Geometry check sheet. Reference: the model listing, model coordinates, mm. A direction names the side the tool comes from. Coordinates: 2 decimals unless noted, no trailing zeros. Write each loop counter-clockwise with the first axis right and the second up, starting at its lowest first coordinate (ties: lowest second). Pieces come first, ordered by that corner, then holes. Notation, with made-up numbers: (-27.75, 75) -> (-1.75, 75) arc R27 ccw to (-1.75, 104) -> close; hole circle Ø10 at (-2.75, 64). An arc over 180 degrees is marked (long way). Answer in a Markdown table with one row per item. Add a question column.
Q1. Section check D-D, the plane x = 0. Count the separate pieces of the cut face and the enclosed holes in it, and give its area (3 significant figures).
Q2. Release check for a two-part mould opening along X. For faces 5 (the face through (-42.15, 250.51, 0.45)), 6 (the face through (0.49, 2.85, -41.99)), 7 (the face through (-1.69, 57.89, 33.87)) record: pulls with the +X half, pulls with the -X half, needs draft (parallel to the pull), parting line crosses it, or undercut.
Q3. Tool access check on faces 1 (the face through (0, 105, 75)), 2 (the face through (0, 22.5, 0)), 3 (the face through (7.067, 56.084, -25.354)), 4 (the face through (42.15, 136.72, 25.51)). Record the directions out of +Z, -Z, +X, -X, +Y, -Y that give a thin tool (end or side, any length) a straight path to the whole face; none if there is none.
Q4. Section check A-A, the plane y = 105. Record the boundary of the cut face in (x, z), and give its area (3 significant figures).
Q5. Thickness scan on line 1 (Y direction, x = 0, z = 32.75); line 2 (Y direction, x = -25, z = -16.5); line 3 (Z direction, x = 9.5, y = 99). Record the ranges inside material, lowest first.
Q6. Section check B-B, the plane y = 170.5. Record the boundary of the cut face in (x, z), and give its area (3 significant figures).
Q7. Gauge pin test, flat ends, axial feed: P1, Ø1, axis at x = -26, y = 241, coming from the -Z side; P2, Ø6, axis at x = -1, y = 132.5, coming from the +Z side; P3, Ø15.5, axis at x = 0, y = 45, coming from the +Z side; P4, Ø10, axis at x = -16, z = -50.5, coming from the -Y side. Record the tip position at first contact, or that the pin passes through.
Q8. Section check C-C, the plane x = -22. Record the boundary of the cut face in (y, z).
```python
from build123d import *

# Parameters (mm, degrees)
SKETCH2_W              = 90
SKETCH2_H              = 90
BOSS_EXTRUDE1_DEPTH    = 270
SKETCH3_W              = 45
SKETCH3_H              = 225
CUT_EXTRUDE1_DEPTH     = 289.140590684
SKETCH4_R              = 25
CRANK_SHAFT_HOLE_DEPTH = 90
SKETCH5_R              = 13
CUT_EXTRUDE3_DEPTH     = 90
CHAMFER1_SIZE          = 3
SKETCH6_R              = 17.5
BOSS_EXTRUDE2_DEPTH    = 30
FILLET1_R              = 10


with BuildPart() as part:
    # Sketch2 → Boss-Extrude1 (new body)
    with BuildSketch(Plane(origin=(0, 0, 0), x_dir=(1, 0, 0), z_dir=(0, 1, 0))):
        Rectangle(SKETCH2_W, SKETCH2_H)
    extrude(amount=BOSS_EXTRUDE1_DEPTH)

    # Sketch3 → Cut-Extrude1 (cut, through all)
    with BuildSketch(Plane(origin=(45, 0, 0), x_dir=(0, 0, -1), z_dir=(1, 0, 0))):
        with Locations((0, 135)):
            Rectangle(SKETCH3_W, SKETCH3_H)
    extrude(amount=-CUT_EXTRUDE1_DEPTH, mode=Mode.SUBTRACT)

    # Sketch4 → Crank shaft hole (cut)
    with BuildSketch(Plane.XY.offset(45)):
        with Locations((0, 170.5)):
            Circle(SKETCH4_R)
    extrude(amount=-CRANK_SHAFT_HOLE_DEPTH, mode=Mode.SUBTRACT)

    # Sketch5 → Cut-Extrude3 (cut)
    with BuildSketch(Plane.XY.offset(45)):
        with Locations((0, 45)):
            Circle(SKETCH5_R)
    extrude(amount=-CUT_EXTRUDE3_DEPTH, mode=Mode.SUBTRACT)

    # Chamfer1
    chamfer1_edges = [part.edges().sort_by_distance(p)[0] for p in [
        (-13, 45, 22.5),
        (-13, 45, -45),
        (-13, 45, -22.5),
        (-13, 45, 45),
    ]]
    chamfer(chamfer1_edges, length=CHAMFER1_SIZE)

    # Sketch6 → Boss-Extrude2 (add)
    with BuildSketch(Plane.XY.offset(45)):
        with Locations(Location((0, 105, 0), (0, 0, 180))):
            Circle(SKETCH6_R)
    boss_extrude2 = extrude(amount=BOSS_EXTRUDE2_DEPTH)

    # Mirror1: Boss-Extrude2 across plane
    add(boss_extrude2.mirror(Plane.XY))

    # Fillet1
    fillet1_edges = [part.edges().sort_by_distance(p)[0] for p in [
        (-45, 270, 0),
        (0, 270, 45),
        (-45, 135, 22.5),
        (-45, 247.5, 0),
        (-45, 135, -22.5),
        (-45, 22.5, 0),
        (45, 135, 22.5),
        (45, 22.5, 0),
        (45, 135, -22.5),
        (45, 247.5, 0),
        (45, 270, 0),
        (0, 0, 45),
        (-45, 0, 0),
        (0, 0, -45),
        (45, 0, 0),
        (45, 135, 45),
        (-45, 135, 45),
        (-45, 135, -45),
        (45, 135, -45),
        (0, 270, -45),
    ]]
    fillet(fillet1_edges, radius=FILLET1_R)


solid = part.part
```
Calculated:
| question | item | result |
|---|---|---|
| 1 | separate pieces | 4 |
| 1 | enclosed holes | 0 |
| 1 | area | 12,700 mm² |
| 2 | face 5 | pulls with the -X half |
| 2 | face 6 | needs draft |
| 2 | face 7 | undercut |
| 3 | face 1 | +Z, +X, -X, +Y, -Y |
| 3 | face 2 | +X, -X |
| 3 | face 3 | none |
| 3 | face 4 | +X |
| 4 | outline | (-45, -35) arc R10 ccw to (-35, -45) -> (-17.5, -45) -> (-17.5, -75) -> (17.5, -75) -> (17.5, -45) -> (35, -45) arc R10 ccw to (45, -35) -> (45, -32.5) arc R10 ccw to (35, -22.5) -> (-35, -22.5) arc R10 ccw to (-45, -32.5) -> close; (-45, 32.5) arc R10 ccw to (-35, 22.5) -> (35, 22.5) arc R10 ccw to (45, 32.5) -> (45, 35) arc R10 ccw to (35, 45) -> (17.5, 45) -> (17.5, 75) -> (-17.5, 75) -> (-17.5, 45) -> (-35, 45) arc R10 ccw to (-45, 35) -> close |
| 4 | area | 5,980 mm² |
| 5 | line 1 | y = 0 to 32, 58 to 145.5, 195.5 to 270 |
| 5 | line 2 | y = 0 to 22.5, 247.5 to 270 |
| 5 | line 3 | z = -75 to -22.5, 22.5 to 75 |
| 6 | outline | (-45, -35) arc R10 ccw to (-35, -45) -> (-25, -45) -> (-25, -22.5) -> (-35, -22.5) arc R10 ccw to (-45, -32.5) -> close; (-45, 32.5) arc R10 ccw to (-35, 22.5) -> (-25, 22.5) -> (-25, 45) -> (-35, 45) arc R10 ccw to (-45, 35) -> close; (25, -45) -> (35, -45) arc R10 ccw to (45, -35) -> (45, -32.5) arc R10 ccw to (35, -22.5) -> (25, -22.5) -> close; (25, 22.5) -> (35, 22.5) arc R10 ccw to (45, 32.5) -> (45, 35) arc R10 ccw to (35, 45) -> (25, 45) -> close |
| 6 | area | 1,630 mm² |
| 7 | P1 | stops at z = -45 |
| 7 | P2 | stops at z = 45 |
| 7 | P3 | passes through |
| 7 | P4 | stops at y = 91.39 |
| 8 | outline | (0, -35) arc R10 ccw to (10, -45) -> (158.63, -45) -> (158.63, -22.5) -> (22.5, -22.5) -> (22.5, 22.5) -> (158.63, 22.5) -> (158.63, 45) -> (10, 45) arc R10 ccw to (0, 35) -> close; (182.37, -45) -> (260, -45) arc R10 ccw to (270, -35) -> (270, 35) arc R10 ccw to (260, 45) -> (182.37, 45) -> (182.37, 22.5) -> (247.5, 22.5) -> (247.5, -22.5) -> (182.37, -22.5) -> close |
